Read the model definition and answer for the solid it produces. Units are mm, in the model's axes. Coordinates: 2 decimals unless noted, no trailing zeros. Write each loop counter-clockwise with the first axis right and the second up, starting at its lowest first coordinate (ties: lowest second). Pieces come first, ordered by that corner, then holes. Notation, with made-up numbers: (10.25, 68.5) -> (15.25, 68.5) arc R25 ccw to (15.25, 96.5) -> close; hole circle Ø3 at (52.5, 80.5). An arc over 180 degrees is marked (long way). Return JSON: item names as keys, results as strings.
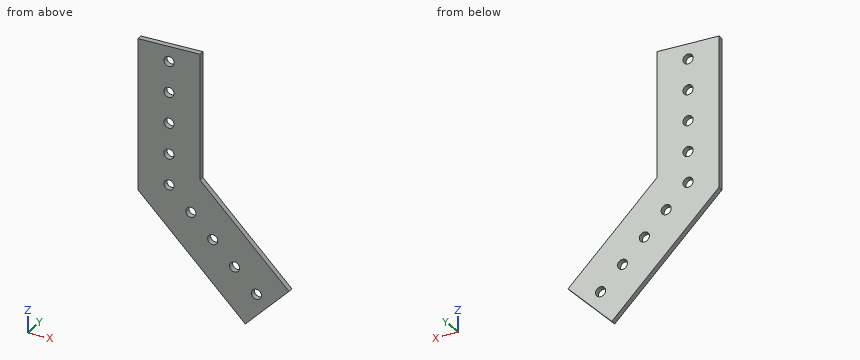
Autodesk Inventor part; units mm, degrees
ref_plane "YZ Plane" through (0, 0, 0) normal (1, 0, 0) x (0, 1, 0)
ref_plane "XZ Plane" through (0, 0, 0) normal (0, 1, 0) x (-1, 0, 0)
ref_plane "XY Plane" through (0, 0, 0) normal (0, 0, 1) x (1, 0, 0)
sketch "Sketch1" plane through (0, 0, 0) normal (0, 1, 0) x (-1, 0, 0)
  line L0 (0, 0) -> (0, -62.2808)
  line L1 (0, -62.2808) -> (-44.0392, -106.32)
  line L2 (-44.0392, -106.32) -> (-61.9997, -88.3595)
  line L3 (-61.9997, -88.3595) -> (-25.4, -51.7598)
  line L4 (-25.4, -51.7598) -> (-25.4, 0)
  line L5 (-25.4, 0) -> (0, 0)
  line L6 (0, -62.2808) -> (-25.4, -51.7598) construction
  dimension "d0" = 62.2808
  dimension "d1" = 25.4
  dimension "d2" = 135
extrude "Extrusion1" add sketch "Sketch1" along normal blind 2.286
sketch "Sketch2" plane through (0, 2.286, 0) normal (0, 1, 0) x (1, 0, 0)
  line L0 (44.0392, 106.32) -> (0, 62.2808)
  line L1 (25.4, 0) -> (25.4, 51.7598)
  line L2 (0, 62.2808) -> (25.4, 51.7598) construction
  point P0 (0, 0)
  point P1 (12.7, 57.0203)
  dimension "d5" = 12.7
hole "Hole1" at (12.7, 2.286, -57.0203) direction (0, -1, 0) diameter 4.1402 end through all
pattern_linear "Rectangular Pattern1" count 5 spacing 12.7 along (0, 0, 1) of "Hole1"
pattern_linear "Rectangular Pattern2" count 5 spacing 12.7 along (0.7071, 0, -0.7071) of "Hole1"
properties part number "135 Gusset"
1. The part is cut by section A-A (y = 1.35). Count the separate pieces of the cut face and the enclosed holes in it, then the cut area to 3 significant figures.
Taken from the geometry:
{"separate pieces": "1", "enclosed holes": "9", "area": "2,780 mm2"}
2. The part is cut by section C-C (z = -79). Determine the outline of the cut face in (x, y), then the cut area to 3 significant figures.
Taken from the geometry:
{"outline": "(16.72, 0) -> (52.64, 0) -> (52.64, 2.29) -> (16.72, 2.29) -> close", "area": "82.1 mm2"}
3. A flat-ended cylindrical pin translates along its axis: pin 1 Ø3.5 at (x, z) = (12.7, -18.92) entering from +Y. Find the tip coordinate at first contact, or state that the pin passes through.
Taken from the geometry:
{"pin 1": "passes through"}
4. The part is cut by section D-D (x = 55). Determine the outline of the cut face in (y, z).
Taken from the geometry:
{"outline": "(0, -95.36) -> (2.29, -95.36) -> (2.29, -81.36) -> (0, -81.36) -> close"}
5. Consider L1, parallel to Z at x = 12, y = 1.9; L2, parallel to X at y = 0.85, z = -4; L3, parallel to Z at x = 12.7, y = 1.6. Determine where each line is inside the solid, lowest interval first.
Taken from the geometry:
{"L1": "z = -74.28 to -58.97, -55.07 to -46.27, -42.37 to -33.57, -29.67 to -20.87, -16.97 to -8.17, -4.27 to 0", "L2": "x = 0 to 25.4", "L3": "z = -74.98 to -59.09, -54.95 to -46.39, -42.25 to -33.69, -29.55 to -20.99, -16.85 to -8.29, -4.15 to 0"}
6. The part is cut by section B-B (x = 12.7). Determine the outline of the cut face in (y, z), then the cut area to 3 significant figures.
Taken from the geometry:
{"outline": "(0, -74.98) -> (2.29, -74.98) -> (2.29, -59.09) -> (0, -59.09) -> close; (0, -54.95) -> (2.29, -54.95) -> (2.29, -46.39) -> (0, -46.39) -> close; (0, -42.25) -> (2.29, -42.25) -> (2.29, -33.69) -> (0, -33.69) -> close; (0, -29.55) -> (2.29, -29.55) -> (2.29, -20.99) -> (0, -20.99) -> close; (0, -16.85) -> (2.29, -16.85) -> (2.29, -8.29) -> (0, -8.29) -> close; (0, -4.15) -> (2.29, -4.15) -> (2.29, 0) -> (0, 0) -> close", "area": "124 mm2"}
